CAD build for the part. Positions are in the model's coordinates, mm. Face numbers are marked on the shaded views. A direction names the side the tool comes from. Give positions to 0.01 mm unless a question says otherwise; leave off trailing zeros. Loops run counter-clockwise (first coordinate to the right, second up) from the corner with the lowest first, then second, coordinate; pieces in that order, holes last. Notation, with made-up numbers: (17.5, -20) -> (68.5, -20) arc R10 cw to (68.5, -8) -> close; hole circle Ø10 at (-31.75, 52). An arc over 180 degrees is marked (long way). Use one line per item in the form item = value.
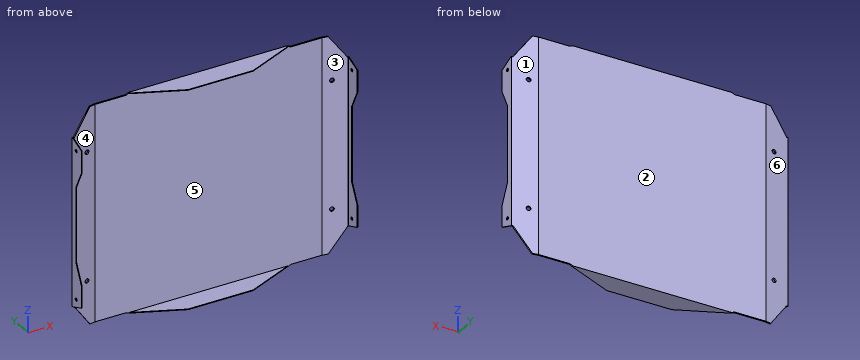
```python
from build123d import *

# Parameters (mm, degrees)
ESQUISSE1_W                  = 416
ESQUISSE1_H                  = 329
BOSS_EXTRU_1_DEPTH           = 33
ENL_V_MAT_EXTRU_1_DEPTH      = 532.400037636
ESQUISSE3_W                  = 2
ESQUISSE3_H                  = 36.5125
ENL_V_MAT_EXTRU_2_DEPTH      = 532.400037636
ENL_V_MAT_EXTRU_3_DEPTH      = 509.456475675
ENL_V_MAT_EXTRU_3_DEPTH_BACK = 509.456475675
ENL_V_MAT_EXTRU_11_DEPTH     = 531.164125531
ENL_V_MAT_EXTRU_4_DEPTH      = 540.111732489
ENL_V_MAT_EXTRU_5_DEPTH      = 540.298629883
ESQUISSE10_W                 = 251.975
ESQUISSE10_H                 = 2.642455338
ENL_V_MAT_EXTRU_6_DEPTH      = 532.400037636
ENL_V_MAT_EXTRU_12_REACH     = 470.566
ESQUISSE18_W                 = 8
ESQUISSE18_H                 = 31
ENL_V_MAT_EXTRU_14_DEPTH     = 600
ESQUISSE20_W                 = 1
ESQUISSE20_H                 = 31
ENL_V_MAT_EXTRU_16_DEPTH     = 466.330172822
ENL_V_MAT_EXTRU_15_DEPTH     = 532.400037636
ESQUISSE21_W                 = 1
ESQUISSE21_H                 = 21.870678089
ENL_V_MAT_EXTRU_17_DEPTH     = 509.456475675
ENL_V_MAT_EXTRU_18_DEPTH     = 532.400037636
D_GAGEMENT_1_41_D            = 6.5278
D_GAGEMENT_1_42_D            = 6.5278
ENL_V_MAT_EXTRU_19_REACH     = 533.4
ESQUISSE27_R                 = 2.38125
ENL_V_MAT_EXTRU_20_REACH     = 533.4
ESQUISSE28_R                 = 2.38125


with BuildPart() as part:
    # Esquisse1 → Boss.-Extru.1 (new body)
    with BuildSketch(Plane(origin=(0, 0, 0), x_dir=(1, 0, 0), z_dir=(0, 1, 0))):
        with Locations((208, 164.5)):
            Rectangle(ESQUISSE1_W, ESQUISSE1_H)
    extrude(amount=-BOSS_EXTRU_1_DEPTH)

    # Esquisse2 → Enlèv. mat.-Extru.1 (cut, through all)
    with BuildSketch(Plane(origin=(0, 0, 0), x_dir=(1, 0, 0), z_dir=(0, 1, 0))):
        Polygon((327.417424305, 0), (332, 2), (416, 2), (416, 0), align=None)
        Polygon((88.582575695, 0), (84, 2), (0, 2), (0, 0), align=None)
        Polygon((88.582575695, 329), (84, 327), (0, 327), (0, 329), align=None)
        Polygon((327.417424305, 329), (332, 327), (416, 327), (416, 329), align=None)
    extrude(amount=-ENL_V_MAT_EXTRU_1_DEPTH, mode=Mode.SUBTRACT)

    # Esquisse3 → Enlèv. mat.-Extru.2 (cut, through all)
    with BuildSketch(Plane(origin=(0, 0, 0), x_dir=(1, 0, 0), z_dir=(0, 1, 0))):
        with Locations((415, 20.25625)):
            Rectangle(ESQUISSE3_W, ESQUISSE3_H)
        with Locations((415, 308.74375)):
            Rectangle(ESQUISSE3_W, ESQUISSE3_H)
        with Locations((1, 308.74375)):
            Rectangle(ESQUISSE3_W, ESQUISSE3_H)
        with Locations((1, 20.25625)):
            Rectangle(ESQUISSE3_W, ESQUISSE3_H)
    extrude(amount=-ENL_V_MAT_EXTRU_2_DEPTH, mode=Mode.SUBTRACT)

    # Esquisse7 → Enlèv. mat.-Extru.3 (cut, two sides: drawn at the far end of the back side and taken through both)
    with BuildSketch(Plane.XY.offset(-38.5125).offset(-ENL_V_MAT_EXTRU_3_DEPTH_BACK)):
        Polygon((416, -6.857544662), (379, 0), (416, 0), align=None)
        Polygon((0, -6.857544662), (37, 0), (0, 0), align=None)
    extrude(amount=ENL_V_MAT_EXTRU_3_DEPTH + ENL_V_MAT_EXTRU_3_DEPTH_BACK, mode=Mode.SUBTRACT)

    # Esquisse15 → Enlèv. mat.-Extru.11 (cut, through all)
    with BuildSketch(Plane(origin=(0, 0, -327), x_dir=(-1, 0, 0), z_dir=(0, 0, -1))):
        Polygon((-84, -33), (-2, -33), (-2, -8.486866573), (-37, -2), (-84, -2), align=None)
        Polygon((-414, -33), (-414, -8.486866573), (-379, -2), (-332, -2), (-332, -33), align=None)
    extrude(amount=-ENL_V_MAT_EXTRU_11_DEPTH, mode=Mode.SUBTRACT)

    # Esquisse8 → Enlèv. mat.-Extru.4 (cut, through all, along a direction that is not the sketch's normal)
    with BuildSketch(Plane(origin=(1.22876211, -6.629807067, 0), x_dir=(0.9832549075639557, 0.1822355254921413, 0), z_dir=(-0.1822355254921413, 0.9832549075639557, 0))):
        Polygon((0.784372276, 38.5125), (27.933724824, 2), (0.784372276, 2), align=None)
        Polygon((0.784372276, 290.4875), (27.933724824, 327), (0.784372276, 327), align=None)
    extrude(amount=-ENL_V_MAT_EXTRU_4_DEPTH, dir=(0, 1, 0), mode=Mode.SUBTRACT)

    # Esquisse9 → Enlèv. mat.-Extru.5 (cut, through all, along a direction that is not the sketch's normal)
    with BuildSketch(Plane(origin=(12.586509179, 67.910726439, 0), x_dir=(0.9832549075639558, -0.18223552549214084, 0), z_dir=(0.18223552549214084, 0.9832549075639558, 0))):
        Polygon((408.24966927, 290.4875), (381.100316723, 327), (408.24966927, 327), align=None)
        Polygon((408.24966927, 38.5125), (381.100316723, 2), (408.24966927, 2), align=None)
    extrude(amount=-ENL_V_MAT_EXTRU_5_DEPTH, dir=(0, 1, 0), mode=Mode.SUBTRACT)

    # Esquisse10 → Enlèv. mat.-Extru.6 (cut, through all)
    with BuildSketch(Plane(origin=(416, 0, 0), x_dir=(0, 0, -1), z_dir=(1, 0, 0))):
        with Locations((164.5, -31.678772331)):
            Rectangle(ESQUISSE10_W, ESQUISSE10_H)
    extrude(amount=-ENL_V_MAT_EXTRU_6_DEPTH, mode=Mode.SUBTRACT)

    # Esquisse16 → Enlèv. mat.-Extru.12 (cut, up to next)
    with BuildSketch(Plane.ZY.offset(-84), mode=Mode.PRIVATE) as enl_v_mat_extru_12_sk1:
        Polygon((-290.4875, -30.357544662), (-290.4875, -33), (-327, -33), (-327, -2), (-2, -2), (-2, -33), (-38.5125, -33), (-38.5125, -30.357544662), align=None)
    enl_v_mat_extru_12_tool1 = extrude(enl_v_mat_extru_12_sk1.sketch, amount=-ENL_V_MAT_EXTRU_12_REACH, mode=Mode.PRIVATE) & part.part
    add(enl_v_mat_extru_12_tool1.solids().sort_by_distance((84, -16.49665, -164.5))[0], mode=Mode.SUBTRACT)

    # Esquisse18 → Enlèv. mat.-Extru.14 (cut)
    with BuildSketch(Plane.XY):
        with Locations((331.417424305, -17.5)):
            Rectangle(ESQUISSE18_W, ESQUISSE18_H)
        with Locations((84.582575695, -17.5)):
            Rectangle(ESQUISSE18_W, ESQUISSE18_H)
    extrude(amount=-ENL_V_MAT_EXTRU_14_DEPTH, mode=Mode.SUBTRACT)

    # Esquisse20 → Enlèv. mat.-Extru.16 (cut, through all)
    with BuildSketch(Plane(origin=(327.417424305, 0, 0), x_dir=(0, 0, -1), z_dir=(1, 0, 0))):
        with Locations((1.5, -17.5)):
            Rectangle(ESQUISSE20_W, ESQUISSE20_H)
        with Locations((327.5, -17.5)):
            Rectangle(ESQUISSE20_W, ESQUISSE20_H)
    extrude(amount=-ENL_V_MAT_EXTRU_16_DEPTH, mode=Mode.SUBTRACT)

    # Esquisse19 → Enlèv. mat.-Extru.15 (cut, through all)
    with BuildSketch(Plane.XY):
        Polygon((88.582575695, -2), (158.997575695, -33), (88.582575695, -33), align=None)
        Polygon((327.417424305, -2), (256.997575695, -33), (327.417424305, -33), align=None)
    extrude(amount=-ENL_V_MAT_EXTRU_15_DEPTH, mode=Mode.SUBTRACT)

    # Esquisse21 → Enlèv. mat.-Extru.17 (cut, through all)
    with BuildSketch(Plane(origin=(0, 0, -290.4875), x_dir=(-1, 0, 0), z_dir=(0, 0, -1))):
        with Locations((-414.5, -19.422205618)):
            Rectangle(ESQUISSE21_W, ESQUISSE21_H)
        with Locations((-1.5, -19.422205618)):
            Rectangle(ESQUISSE21_W, ESQUISSE21_H)
    extrude(amount=-ENL_V_MAT_EXTRU_17_DEPTH, mode=Mode.SUBTRACT)

    # Esquisse22 → Enlèv. mat.-Extru.18 (cut, through all)
    with BuildSketch(Plane(origin=(416, 0, 0), x_dir=(0, 0, -1), z_dir=(1, 0, 0))):
        Polygon((38.5125, -8.486866573), (47.110374149, -30.357544662), (38.5125, -30.357544662), align=None)
        Polygon((290.4875, -8.486866573), (281.889625851, -30.357544662), (290.4875, -30.357544662), align=None)
        Polygon((80.110374149, -30.357544662), (108.145374149, -16.357544662), (220.645374149, -16.357544662), (248.889625851, -30.357544662), align=None)
    extrude(amount=-ENL_V_MAT_EXTRU_18_DEPTH, mode=Mode.SUBTRACT)

    # Dégagement 1/41 (through all)
    with Locations(Plane(origin=(12.586509179, 67.910726439, 0), x_dir=(0.9832549075639558, -0.18223552549214084, 0), z_dir=(0.18223552549214084, 0.9832549075639558, 0))):
        with Locations((386.653609967, 68.25), (386.653609967, 260.75)):
            Hole(D_GAGEMENT_1_41_D / 2)

    # Dégagement 1/42 (through all)
    with Locations(Plane(origin=(1.22876211, -6.629807067, 0), x_dir=(0.9832549075639557, 0.18223552549214128, 0), z_dir=(-0.1822355254921413, 0.9832549075639558, 0))):
        with Locations((22.38043158, 68.25), (22.38043158, 260.75)):
            Hole(D_GAGEMENT_1_42_D / 2)

    # Esquisse27 → Enlèv. mat.-Extru.19 (cut, up to next)
    with BuildSketch(Plane.ZY, mode=Mode.PRIVATE) as enl_v_mat_extru_19_sk1:
        with Locations((-275.4875, -16.857544662)):
            Circle(ESQUISSE27_R)
    enl_v_mat_extru_19_tool1 = extrude(enl_v_mat_extru_19_sk1.sketch, amount=-ENL_V_MAT_EXTRU_19_REACH, mode=Mode.PRIVATE) & part.part
    # Esquisse27 → Enlèv. mat.-Extru.19 (cut, up to next)
    with BuildSketch(Plane.ZY, mode=Mode.PRIVATE) as enl_v_mat_extru_19_sk2:
        with Locations((-53.5125, -16.857544662)):
            Circle(ESQUISSE27_R)
    enl_v_mat_extru_19_tool2 = extrude(enl_v_mat_extru_19_sk2.sketch, amount=-ENL_V_MAT_EXTRU_19_REACH, mode=Mode.PRIVATE) & part.part
    add(enl_v_mat_extru_19_tool1.solids().sort_by_distance((0, -16.857545, -275.4875))[0], mode=Mode.SUBTRACT)
    add(enl_v_mat_extru_19_tool2.solids().sort_by_distance((0, -16.857545, -53.5125))[0], mode=Mode.SUBTRACT)

    # Esquisse28 → Enlèv. mat.-Extru.20 (cut, up to next)
    with BuildSketch(Plane(origin=(416, 0, 0), x_dir=(0, 0, -1), z_dir=(1, 0, 0)), mode=Mode.PRIVATE) as enl_v_mat_extru_20_sk1:
        with Locations(Location((53.5125, -16.857544662, 0), (0, 0, 180))):
            Circle(ESQUISSE28_R)
    enl_v_mat_extru_20_tool1 = extrude(enl_v_mat_extru_20_sk1.sketch, amount=-ENL_V_MAT_EXTRU_20_REACH, mode=Mode.PRIVATE) & part.part
    # Esquisse28 → Enlèv. mat.-Extru.20 (cut, up to next)
    with BuildSketch(Plane(origin=(416, 0, 0), x_dir=(0, 0, -1), z_dir=(1, 0, 0)), mode=Mode.PRIVATE) as enl_v_mat_extru_20_sk2:
        with Locations(Location((275.4875, -16.857544662, 0), (0, 0, 180))):
            Circle(ESQUISSE28_R)
    enl_v_mat_extru_20_tool2 = extrude(enl_v_mat_extru_20_sk2.sketch, amount=-ENL_V_MAT_EXTRU_20_REACH, mode=Mode.PRIVATE) & part.part
    add(enl_v_mat_extru_20_tool1.solids().sort_by_distance((416, -16.857545, -53.5125))[0], mode=Mode.SUBTRACT)
    add(enl_v_mat_extru_20_tool2.solids().sort_by_distance((416, -16.857545, -275.4875))[0], mode=Mode.SUBTRACT)


solid = part.part
```
1. Drop flat-ended pins along their axis: P1, Ø5, axis at x = 169.5, z = -241, coming from the +Y side; P2, Ø1.1, axis at x = 0.5, z = -55.5, coming from the -Y side; P3, Ø4, axis at x = 358, y = -2, coming from the -Z side; P4, Ø8, axis at x = 272, z = -167, coming from the -Y side. Give the stop position or say it passes through.
Result sheet:
P1 = 0
P2 = -30.36
P3 = -327
P4 = -2
2. Cut at D-D, the plane x = 374.5. Write the cut outline in (y, z).
Result sheet:
outline = (-2, -327) -> (0, -327) -> (0, -2) -> (-2, -2) -> close
3. Tool access for the marked faces 4, 5 and 6: list every direction of +Z, -Z, +X, -X, +Y, -Y with a clear straight run to the whole face (end or side of a thin tool).
Result sheet:
face_4 = +Z, -Z, -Y
face_5 = -Y
face_6 = +Z, -Z, -X, +Y
4. Drill centre lines: line 1 (X direction, y = -18, z = -66.5); line 2 (Z direction, x = 231.5, y = -3); line 3 (Y direction, x = 228.5, z = -72.5). Where is each one in solid material? Low to high.
Result sheet:
line_1 = 0 to 1, 415 to 416
line_2 = -329 to -328, -1 to 0
line_3 = -2 to 0
5. Cut at C-C, the plane z = -211. Write the cut outline in (x, y).
Result sheet:
outline = (0, -16.36) -> (1, -16.36) -> (1, -8.49) -> (2, -8.49) -> (37, -2) -> (379, -2) -> (414, -8.49) -> (415, -8.49) -> (415, -16.36) -> (416, -16.36) -> (416, -6.86) -> (379, 0) -> (37, 0) -> (0, -6.86) -> close
6. Cut at B-B, the plane x = 175. Write the cut outline in (y, z).
Result sheet:
outline = (-33, -329) -> (0, -329) -> (0, 0) -> (-33, 0) -> (-33, -1) -> (-2, -1) -> (-2, -328) -> (-33, -328) -> close
7. Mould opens along X. For the marked faces 1, 2 and 3 say: pulls with the +X half, pulls with the -X half, needs draft (parallel to the pull), parting line crosses it, or undercut.
Result sheet:
face_1 = pulls with the +X half
face_2 = needs draft
face_3 = undercut
8. Cut at A-A, the plane y = -24.5. Write the cut outline in (x, z), then the cut area to 3 significant figures.
Result sheet:
outline = (0, -284.19) -> (1, -284.19) -> (1, -237.07) -> (0, -237.07) -> close; (0, -91.84) -> (1, -91.84) -> (1, -44.81) -> (0, -44.81) -> close; (139.69, -329) -> (276.31, -329) -> (276.31, -328) -> (139.69, -328) -> close; (139.69, -1) -> (276.31, -1) -> (276.31, 0) -> (139.69, 0) -> close; (415, -284.19) -> (416, -284.19) -> (416, -237.07) -> (415, -237.07) -> close; (415, -91.84) -> (416, -91.84) -> (416, -44.81) -> (415, -44.81) -> close
area = 462 mm^2
